from build123d import *

# Parameters (mm, degrees)
SKETCH3_W          = 12
SKETCH3_H          = 1.5
CHAMFER1_SIZE      = 0.45
CUT_EXTRUDE1_DEPTH = 1.19


with BuildPart() as part:
    # Sketch3 → Revolve1 (revolve)
    with BuildSketch(Plane(origin=(0, 0, 0), x_dir=(0, 0, -1), z_dir=(1, 0, 0))):
        with Locations((0, 0.75)):
            Rectangle(SKETCH3_W, SKETCH3_H)
    revolve(axis=Axis((0, 0, -6), (0, 0, 1)))

    # Chamfer1
    chamfer1_edges = [part.edges().sort_by_distance(p)[0] for p in [
        (0, -1.5, -6),
    ]]
    chamfer(chamfer1_edges, length=CHAMFER1_SIZE)

    # Sketch6 → Revolve2 (revolve)
    with BuildSketch(Plane(origin=(0, 0, 0), x_dir=(0, 0, -1), z_dir=(1, 0, 0))):
        Polygon((-6, 3), (-5.8, 3), (-4.3, 1.5), (-4.3, 0), (-6, 0), align=None)
    revolve(axis=Axis((0, 0, -6), (0, 0, 1)))

    # Sketch8 → Cut-Extrude1 (cut)
    with BuildSketch(Plane.XY.offset(6)):
        Polygon((0, 1.154700538), (-1, 0.577350269), (-1, -0.577350269), (0, -1.154700538), (1, -0.577350269), (1, 0.577350269), align=None)
    extrude(amount=-CUT_EXTRUDE1_DEPTH, mode=Mode.SUBTRACT)

    # Cut-Extrude2 cone 1 section (through the dimple's axis) → Cut-Extrude2 (revolve, cut)
    with BuildSketch(Plane(origin=(0, 0, 6), x_dir=(0, -1, 0), z_dir=(1, 0, 0))):
        Polygon((0, 0), (1.154700538, 0), (0, 1.154700538), align=None)
    revolve(axis=Axis((0, 0, 6), (0, 0, -1)), mode=Mode.SUBTRACT)


solid = part.part
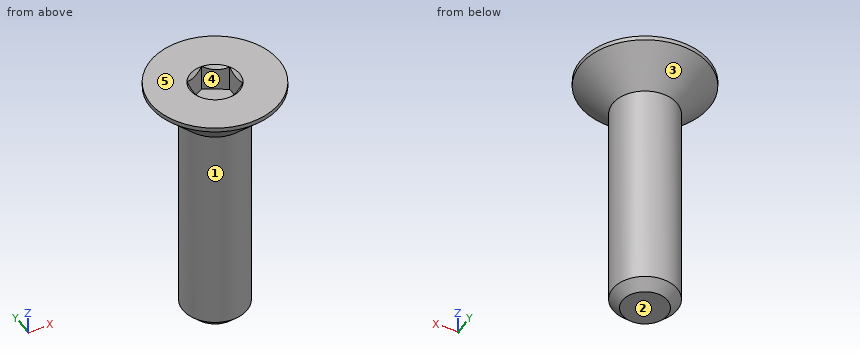
Geometry: final body of the model. Coordinates: model frame, mm. Face numbers are marked on the shaded views. A direction names the side the tool comes from. Give positions to 0.01 mm unless a question says otherwise; leave off trailing zeros. Write each loop counter-clockwise with the first axis right and the second up, starting at its lowest first coordinate (ties: lowest second). Pieces come first, ordered by that corner, then holes. Notation, with made-up numbers: (-15.5, 78) -> (18.5, 78) arc R17 ccw to (18.5, 97) -> close; hole circle Ø4 at (63.5, 10). An arc over 180 degrees is marked (long way). Answer as a JSON object with one key per item and string values.
1. Cut plane A-A on y = 0. Output: boundary loops of the cut face in (x, z).
Ans:
{"outline": "(-3, 5.8) -> (-1.5, 4.3) -> (-1.5, -5.55) -> (-1.05, -6) -> (1.05, -6) -> (1.5, -5.55) -> (1.5, 4.3) -> (3, 5.8) -> (3, 6) -> (1.15, 6) -> (1, 5.85) -> (1, 4.81) -> (-1, 4.81) -> (-1, 5.85) -> (-1.15, 6) -> (-3, 6) -> close"}
2. Mould query, pull axis Y, two halves, no side actions, for the marked faces 3, 4 and 5. Classes: pulls with the +Y half, pulls with the -Y half, needs draft (parallel to the pull), parting line crosses it, or undercut.
Ans:
{"face 3": "parting line crosses it", "face 4": "undercut", "face 5": "needs draft"}
3. Ray query, probe 1 along Z at (x, y) = (-0.1, 0.85); probe 2 along Z at (x, y) = (0.3, 1.35); probe 3 along X at (y, z) = (0.1, 0.75). Return the intervals inside material, ascending. Write a range as from..to.
Ans:
{"probe 1": "z = -6..4.81", "probe 2": "z = -5.67..6", "probe 3": "x = -1.5..1.5"}
4. Cut plane B-B on z = -3.5. Output: boundary loops of the cut face in (x, y).
Ans:
{"outline": "circle Ø3 at (0, 0)"}
5. Contact query for flat-ended pins moving along their axis: pin 1 (3 mm diameter, centred on y = -0.5, z = -3.5, fed in from +X); pin 2 (1 mm diameter, centred on y = 1.5, z = 2.5, fed in from +X); pin 3 (1 mm diameter, centred on x = 0, z = -4.5, fed in from -Y). Output: stop coordinate, or through.
Ans:
{"pin 1": "stops at x = 1.5", "pin 2": "stops at x = 1.12", "pin 3": "stops at y = -1.5"}
6. Access query for the marked faces 1 and 2. Directions: +Z, -Z, +X, -X, +Y, -Y. A direction counts if a zero-diameter tool reaches every point of the face in a straight line with its end or side. Return the directions, or none.
Ans:
{"face 1": "-Z", "face 2": "-Z, +X, -X, +Y, -Y"}
